Source: CAD feature listing. Evaluate the final solid. Frame: model axes, mm. Give positions to 0.01 mm unless a question says otherwise; leave off trailing zeros. Loops run counter-clockwise (first coordinate to the right, second up) from the corner with the lowest first, then second, coordinate; pieces in that order, holes last. Notation, with made-up numbers: (-8, -21) -> (42, -21) arc R30 ccw to (42, 9) -> close; hole circle Ø2 at (-35.75, 27). An arc over 180 degrees is marked (long way). Return JSON: item names as keys, results as strings. Group by question number.
(1) Cut plane A-A on z = 4.5. Return loops of the section in (x, y), then the cut area to 3 significant figures.
(2) Ray query, line 1 (Y direction, x = 0, z = 4.75); line 2 (X direction, y = -0.5, z = 2.5); line 3 (X direction, y = -3, z = 1.75). Return the intervals inside material, ascending. Write a range as from..to.
(3) Draft query along X for faces 1 (the face through (3.358, 5.849, 5.956)), 2 (the face through (-0.867, -3.905, 3.057)), 3 (the face through (-5.6, 3.3, 3.1)), 4 (the face through (3, 3, 6.2)). Return one class per face: released by +X, released by -X, zero draft, split by the parting line, or undercut.
(4) Pin query (flat end, axial travel): pin 1 (1 mm diameter, centred on y = -3.5, z = 5, fed in from -X); pin 2 (1 mm diameter, centred on y = 2.5, z = 3, fed in from +X); pin 3 (1 mm diameter, centred on y = 4, z = 5, fed in from +X). Return the tip coordinate at first contact, or that it passes through.
(5) Cut plane B-B on z = 5.5. Return loops of the section in (x, y).
```python
from build123d import *

# Parameters (mm, degrees)
ESBO_O1_R                = 4
RESSALTO_EXTRUS_O1_DEPTH = 6.2
ESBO_O2_OUTSIDE_W        = 33.572
ESBO_O2_OUTSIDE_H        = 31.56
ESBO_O2_OUTSIDE_R        = 6.5
CORTE_EXTRUS_O1_DEPTH    = 6.2
CORTE_EXTRUS_O1_TAPER    = 45
ESBO_O3_OUTSIDE_W        = 33.572
ESBO_O3_OUTSIDE_H        = 31.56
ESBO_O3_OUTSIDE_R        = 6.5
CORTE_EXTRUS_O2_DEPTH    = 6.2
CORTE_EXTRUS_O2_TAPER    = 45


with BuildPart() as part:
    # Esboço1 → Ressalto-extrusão1 (new body)
    with BuildSketch(Plane.XY):
        Polygon((3.75277675, -6.5), (7.505553499, 0), (3.75277675, 6.5), (-3.75277675, 6.5), (-7.505553499, 0), (-3.75277675, -6.5), align=None)
        Circle(ESBO_O1_R, mode=Mode.SUBTRACT)
    extrude(amount=RESSALTO_EXTRUS_O1_DEPTH)

    # Esboço2 outside → Corte-extrusão1 (cut)
    with BuildSketch(Plane.XY.offset(6.2)):
        Rectangle(ESBO_O2_OUTSIDE_W, ESBO_O2_OUTSIDE_H)
        Circle(ESBO_O2_OUTSIDE_R, mode=Mode.SUBTRACT)
    extrude(amount=-CORTE_EXTRUS_O1_DEPTH, taper=CORTE_EXTRUS_O1_TAPER, mode=Mode.SUBTRACT)

    # Esboço3 outside → Corte-extrusão2 (cut)
    with BuildSketch(Plane(origin=(0, 0, 0), x_dir=(-1, 0, 0), z_dir=(0, 0, -1))):
        Rectangle(ESBO_O3_OUTSIDE_W, ESBO_O3_OUTSIDE_H)
        Circle(ESBO_O3_OUTSIDE_R, mode=Mode.SUBTRACT)
    extrude(amount=-CORTE_EXTRUS_O2_DEPTH, taper=CORTE_EXTRUS_O2_TAPER, mode=Mode.SUBTRACT)


solid = part.part
```
Answers:
{
 "1": {"outline": "(-7.51, 0) -> (-3.75, -6.5) -> (3.75, -6.5) -> (7.51, 0) -> (3.75, 6.5) -> (-3.75, 6.5) -> close; hole circle Ø8 at (0, 0)", "area": "96.1 mm²"},
 "2": {"line 1": "-6.5..-4, 4..6.5", "line 2": "-7.22..-3.97, 3.97..7.22", "line 3": "-5.77..-2.65, 2.65..5.77"},
 "3": {"face 1": "released by +X", "face 2": "undercut", "face 3": "released by -X", "face 4": "zero draft"},
 "4": {"pin 1": "x = -5.77", "pin 2": "x = 6.35", "pin 3": "x = 5.48"},
 "5": {"outline": "(-7.18, -0.57) -> (-4.08, -5.93) arc R7.2 ccw to (-3.1, -6.5) -> (3.1, -6.5) arc R7.2 ccw to (4.08, -5.93) -> (7.18, -0.57) arc R7.2 ccw to (7.18, 0.57) -> (4.08, 5.93) arc R7.2 ccw to (3.1, 6.5) -> (-3.1, 6.5) arc R7.2 ccw to (-4.08, 5.93) -> (-7.18, 0.57) arc R7.2 ccw to start; hole circle Ø8 at (0, 0)"}
}
